The model under review builds one solid part; all positions refer to its coordinate system, in mm. A direction names the side the tool comes from. Coordinates: 2 decimals unless noted, no trailing zeros. Order: outer loops, then holes, each group sorted by start corner. A loop starts at its lowest first (then second) coordinate and runs counter-clockwise, first axis right, second up. Notation, with made-up numbers: (13.25, 88.25) -> (38.25, 88.25) arc R33 ccw to (38.25, 119.25) -> close; hole circle Ø7 at (-16.75, 28.5). An arc over 180 degrees is marked (long way). Answer as CSV lines item,"result". Start each with the question number.
from build123d import *

# Parameters (mm, degrees)
BOSS_EXTRUDE1_DEPTH = 12.7
CUT_EXTRUDE1_DEPTH  = 12.7
CUT_EXTRUDE2_DEPTH  = 2.54


with BuildPart() as part:
    # Sketch1 → Boss-Extrude1 (new body)
    with BuildSketch(Plane(origin=(0, 0, 0), x_dir=(1, 0, 0), z_dir=(0, 1, 0))):
        Polygon((-10.842199515, -5.384904617), (0.613239188, 0.098062109), (4.836414625, 12.07532345), (-0.6465521, 23.530762153), (-12.623813441, 27.75393759), (-24.079252145, 22.270970865), (-28.302427581, 10.293709523), (-22.819460856, -1.16172918), align=None)
    extrude(amount=BOSS_EXTRUDE1_DEPTH)

    # Sketch2 → Cut-Extrude1 (cut)
    with BuildSketch(Plane(origin=(0.514674893, 0, 0.18147407), x_dir=(0.33253349893190465, 0, -0.9430914441813716), z_dir=(0.9430914441813716, 0, 0.33253349893190465))):
        with BuildLine():
            ThreePointArc((9.236420315, 6.400016207), (9.043074328, 7.372032125), (8.49247154, 8.196067431))
            Line((8.49247154, 8.196067431), (6.646404109, 6.35))
            Line((6.646404109, 6.35), (8.441758775, 4.554645333))
            ThreePointArc((8.441758775, 4.554645333), (9.029311192, 5.395416707), (9.236420315, 6.400016207))
        make_face()
        with BuildLine():
            Line((6.646404109, 6.35), (8.49247154, 8.196067431))
            ThreePointArc((8.49247154, 8.196067431), (6.661050087, 8.939769925), (4.851049442, 8.145354667))
            Line((4.851049442, 8.145354667), (6.646404109, 6.35))
        make_face()
        with BuildLine():
            Line((8.441758775, 4.554645333), (6.646404109, 6.35))
            Line((6.646404109, 6.35), (4.900369091, 4.603964983))
            ThreePointArc((4.900369091, 4.603964983), (6.661050087, 3.860262489), (8.441758775, 4.554645333))
        make_face()
        with BuildLine():
            Line((4.900369091, 4.603964983), (6.646404109, 6.35))
            Line((6.646404109, 6.35), (4.851049442, 8.145354667))
            ThreePointArc((4.851049442, 8.145354667), (4.156666598, 6.364645978), (4.900369091, 4.603964983))
        make_face()
    extrude(amount=-CUT_EXTRUDE1_DEPTH, mode=Mode.SUBTRACT)

    # Sketch3 → Cut-Extrude2 (cut)
    with BuildSketch(Plane.XZ):
        with BuildLine():
            ThreePointArc((-14.953750816, -11.01136249), (-13.141781341, -14.030145133), (-9.65800947, -13.520620278))
            Line((-9.65800947, -13.520620278), (-11.762472687, -11.182932321))
            Line((-11.762472687, -11.182932321), (-14.953750816, -11.01136249))
        make_face()
        with BuildLine():
            Line((-11.762472687, -11.182932321), (-9.65800947, -13.520620278))
            ThreePointArc((-9.65800947, -13.520620278), (-8.922077868, -12.53930026), (-8.613045297, -11.352252168))
            Line((-8.613045297, -11.352252168), (-11.762472687, -11.182932321))
        make_face()
        with BuildLine():
            Line((-14.953750816, -11.01136249), (-11.762472687, -11.182932321))
            Line((-11.762472687, -11.182932321), (-13.906542304, -8.80124863))
            ThreePointArc((-13.906542304, -8.80124863), (-14.651486566, -9.801429), (-14.953750816, -11.01136249))
        make_face()
        with BuildLine():
            Line((-13.906542304, -8.80124863), (-11.762472687, -11.182932321))
            Line((-11.762472687, -11.182932321), (-8.613045297, -11.352252168))
            ThreePointArc((-8.613045297, -11.352252168), (-8.608718567, -11.256636797), (-8.607275887, -11.160934454))
            ThreePointArc((-8.607275887, -11.160934454), (-10.490749827, -8.260488723), (-13.906542304, -8.80124863))
        make_face()
    extrude(amount=-CUT_EXTRUDE2_DEPTH, mode=Mode.SUBTRACT)


solid = part.part
1) Insertion check: pin 1 Ø1.5 at (x, y) = (-6, 8.5) entering from -Z; pin 2 Ø3 at (y, z) = (2.5, -7) entering from -X; pin 3 Ø1.5 at (x, y) = (-6.5, 9) entering from -Z. Each pin has a flat end and moves straight along its axis. Give the tip position at first contact, or say it passes through.
2) Consider section D-D (z = -1). Give the boundary of the cut face in (x, y), plus the area to 3 significant figures.
3) Wall thickness on L1, parallel to Z at x = -3.5, y = 7.5; L2, parallel to Z at x = -2.5, y = 7.75; L3, parallel to Z at x = -15.5, y = 12: over which ranges is each line inside the solid? List them lowest first. Write a range as [from, to].
4) Consider section A-A (y = 1.5). Give the boundary of the cut face in (x, z) (3 decimals), plus the area to 3 significant figures.
5) Consider section C-C (x = -13.5). Give the boundary of the cut face in (y, z), plus the area to 3 significant figures.
6) Consider section B-B (y = 5.25). Give the boundary of the cut face in (x, z).
7) Mouldability with a two-part tool opening along X and no side actions: class faces 1 (the face through (-9.25, 6.44, -10.32)), 2 (the face through (-12, 12.7, -11)), 3 (the face through (-18.27, 6.26, -25.05)) as released by +X, released by -X, zero draft, split by the parting line, or undercut.
8) Tool access review of faces 4 (the face through (-25.6, 6.26, -4.65)), 5 (the face through (-12, 2.54, -11)): name each direction out of +Z, -Z, +X, -X, +Y, -Y from which nothing blocks a thin tool from reaching the whole face with its end or side.
Result:
1,pin 1,"z = -25.68"
1,pin 2,"x = -27.44"
1,pin 3,"z = -25.86"
2,outline,"(-23.85, 0) -> (0.93, 0) -> (0.93, 12.7) -> (-23.85, 12.7) -> close"
2,area,"315 mm2"
3,L1,"[-24.54, -10.76], [-5.91, 1.87]"
3,L2,"[-24.18, -10.26], [-5.7, 1.39]"
3,L3,"[-26.38, 3.74]"
4,outline,"(-28.302, -10.294) -> (-24.079, -22.271) -> (-12.624, -27.754) -> (-0.647, -23.531) -> (4.836, -12.075) -> (0.613, -0.098) -> (-10.842, 5.385) -> (-22.819, 1.162) -> close; hole circle Ø6.35 at (-11.782, -11.161)"
4,area,"747 mm2"
5,outline,"(0, -27.33) -> (12.7, -27.33) -> (12.7, 4.45) -> (0, 4.45) -> (0, -8.49) -> (2.54, -8.49) -> (2.54, -13.83) -> (0, -13.83) -> close"
5,area,"390 mm2"
6,outline,"(-28.3, -10.29) -> (-24.08, -22.27) -> (-12.62, -27.75) -> (-0.65, -23.53) -> (4.84, -12.08) -> (3.49, -8.27) -> (-8.48, -12.49) -> (-9.99, -8.22) -> (1.99, -4) -> (0.61, -0.1) -> (-10.84, 5.38) -> (-22.82, 1.16) -> close"
7,face 1,"undercut"
7,face 2,"zero draft"
7,face 3,"released by -X"
8,face 4,"+Z, -X, +Y, -Y"
8,face 5,"-Y"
